Can you work these out from the model? Positions are in its coordinate system, mm. Face numbers are marked on the shaded views. A direction names the side the tool comes from. Give positions to 0.01 mm unless a question says otherwise; leave off trailing zeros. Write each loop counter-clockwise with the first axis right and the second up, starting at its lowest first coordinate (ties: lowest second). Pieces come first, ordered by that corner, then holes.
1. Suppose I cut it at A-A (y = -44.5). Please give me the cut outline in (x, z).
2. If I drill on probe 1 along Y at (x, z) = (30.8, -0.35); probe 2 along Y at (x, z) = (-77.5, 0.2); probe 3 along X at (y, z) = (38, 16), over which ranges is the centre line in solid material (lowest first)?
3. On a 3-axis mill with a long thin cutter (end or side, diameter ignored), from which of +Z, -Z, +X, -X, +Y, -Y can I reach the whole of each face in a straight line? I mean the marked faces 1, 2, 3 and 4. Say none if no direction works.
4. Suppose I cut it at D-D (x = 39.5). Please give me the cut outline in (y, z), and give its area (3 significant figures).
5. I'm going to push flat-ended pins straight in: pin 1 (1.5 mm diameter, centred on y = 14.5, z = 11.5, fed in from -X); pin 2 (10.5 mm diameter, centred on x = -79, y = -11.5, fed in from +Z); pin 3 (8 mm diameter, centred on x = -78, z = 6.5, fed in from +Y). Where does each tip first touch, or does it pass through?
6. Suppose I cut it at C-C (y = 28.5). Please give me the cut outline in (x, z).
7. Suppose I cut it at B-B (x = -62). Please give me the cut outline in (y, z).
```python
from build123d import *

# Parameters (mm, degrees)
F1_W     = 160
F1_H     = 100
F1_R     = 1.75
F1_R_2   = 2
F2_DEPTH = 0.6
F3_W     = 54
F3_H     = 108
F4_DEPTH = 16
F5_W     = 40
F5_H     = 21
F6_DEPTH = 10


with BuildPart() as f2:
    # F1 (on Top) → F2 (new body, symmetric)
    with BuildSketch(Plane.XY):
        Rectangle(F1_W, F1_H)
        with Locations((-77.5, -44.5)):
            Circle(F1_R, mode=Mode.SUBTRACT)
        with Locations((30.8, -36)):
            Circle(F1_R_2, mode=Mode.SUBTRACT)
        with Locations((66.1, -38.8)):
            Circle(F1_R_2, mode=Mode.SUBTRACT)
        with Locations((-77.5, 44.5)):
            Circle(F1_R, mode=Mode.SUBTRACT)
        with Locations((31.2, 35.8)):
            Circle(F1_R_2, mode=Mode.SUBTRACT)
        with Locations((66.95, 37.8)):
            Circle(F1_R_2, mode=Mode.SUBTRACT)
    extrude(amount=F2_DEPTH, both=True)

    # F3 (on face) → F4 (join)
    with BuildSketch(Plane.XY.offset(0.6)):
        with Locations((-28, -6)):
            Rectangle(F3_W, F3_H)
    extrude(amount=F4_DEPTH)

    # F5 (on face) → F6 (join)
    with BuildSketch(Plane.XY.offset(0.6)):
        with Locations((-80, -6.5)):
            Rectangle(F5_W, F5_H)
    extrude(amount=F6_DEPTH)


solid = f2.part
```
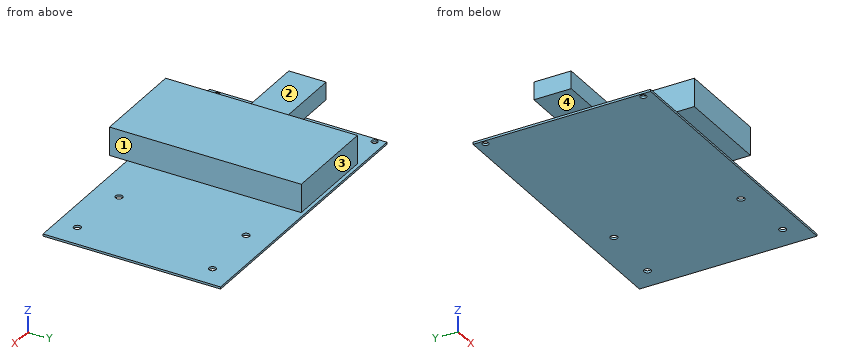
Checks:
1. outline: (-80, -0.6) - (-79.25, -0.6) - (-79.25, 0.6) - (-80, 0.6) - close; (-75.75, -0.6) - (80, -0.6) - (80, 0.6) - (-1, 0.6) - (-1, 16.6) - (-55, 16.6) - (-55, 0.6) - (-75.75, 0.6) - close
2. probe 1: y = -50 to -38, -34 to 33.84, 37.76 to 50
2. probe 2: y = -50 to -46.25, -42.75 to 42.75, 46.25 to 50
2. probe 3: x = -55 to -1
3. face 1: +Z, +X, +Y, -Y
3. face 2: +Z, -X, +Y, -Y
3. face 3: +Z, +X, -X, +Y
3. face 4: -Z, -X, +Y, -Y
4. outline: (-50, -0.6) - (50, -0.6) - (50, 0.6) - (-50, 0.6) - close
4. area: 120 mm2
5. pin 1: stops at x = -55
5. pin 2: stops at z = 10.6
5. pin 3: stops at y = 4
6. outline: (-80, -0.6) - (80, -0.6) - (80, 0.6) - (-1, 0.6) - (-1, 16.6) - (-55, 16.6) - (-55, 0.6) - (-80, 0.6) - close
7. outline: (-50, -0.6) - (50, -0.6) - (50, 0.6) - (4, 0.6) - (4, 10.6) - (-17, 10.6) - (-17, 0.6) - (-50, 0.6) - close
